```python
from build123d import *

# Parameters (mm, degrees)
EXTRUDE_1_DEPTH = 50
SHELL_1_T       = -5
EXTRUDE_3_DEPTH = 45


with BuildPart() as part:
    # 스케치1 → 보스-돌출1 (new body)
    with BuildSketch(Plane(origin=(0, 0, 0), x_dir=(1, 0, 0), z_dir=(0, 1, 0))):
        with BuildLine():
            Line((10, 0), (270, 0))
            ThreePointArc((270, 0), (277.071067812, 2.928932188), (280, 10))
            Line((280, 10), (280, 220))
            ThreePointArc((280, 220), (277.071067812, 227.071067812), (270, 230))
            Line((270, 230), (10, 230))
            ThreePointArc((10, 230), (2.928932188, 227.071067812), (0, 220))
            Line((0, 220), (0, 10))
            ThreePointArc((0, 10), (2.928932188, 2.928932188), (10, 0))
        make_face()
    extrude(amount=EXTRUDE_1_DEPTH)

    # 쉘1
    shell_1_openings = [part.faces().sort_by_distance(p)[0] for p in [
        (140, 50, -115),
    ]]
    offset(amount=SHELL_1_T, openings=shell_1_openings, kind=Kind.INTERSECTION)

    # 스케치4 → 보스-돌출3 (add)
    with BuildSketch(Plane(origin=(0, 5, 0), x_dir=(1, 0, 0), z_dir=(0, 1, 0))):
        Polygon((5, 117.5), (5, 112.5), (92.5, 112.5), (92.5, 5), (97.5, 5), (97.5, 112.5), (180, 112.5), (180, 5), (185, 5), (185, 112.5), (275, 112.5), (275, 117.5), (185, 117.5), (185, 225), (180, 225), (180, 117.5), (97.5, 117.5), (97.5, 225), (92.5, 225), (92.5, 117.5), align=None)
    extrude(amount=EXTRUDE_3_DEPTH)


solid = part.part
```
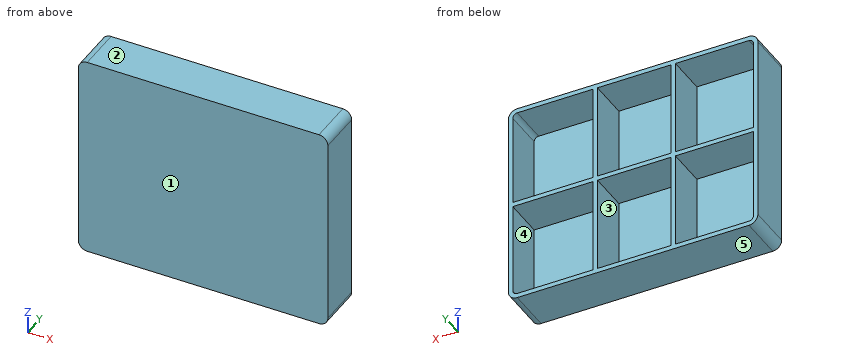
Could you check a few things on this model? Use its own coordinates, in mm. Face numbers are marked on the shaded views. A direction names the side the tool comes from. Round coordinates to 2 decimals unless told otherwise and drop trailing zeros. Order: outer loops, then holes, each group sorted by start corner. A loop starts at its lowest first (then second) coordinate and runs counter-clockwise, first axis right, second up. Notation, with made-up numbers: (-38.5, 23) -> (13.5, 23) arc R12 ccw to (13.5, 37) -> close; hole circle Ø1 at (29, 55). An arc over 180 degrees is marked (long way). One line per question, with ' | ' between items.
Q1. Which directions (+Z, -Z, +X, -X, +Y, -Y) give clear straight access to the entire face, cutting with the end or side of a thin tool? Please do the marked faces 4 and 5.
Computed values:
face 4: +Y | face 5: -Z, +X, -X, +Y, -Y
Q2. If I drill on line 1 (X direction, y = 13, z = -218); line 2 (Z direction, x = 176.5, y = 22.5); line 3 (Y direction, x = 130.5, z = -208), over which ranges is the centre line in solid material (lowest first)? Write a range as from..to.
Computed values:
line 1: 0..5, 92.5..97.5, 180..185, 275..280 | line 2: -230..-225, -117.5..-112.5, -5..0 | line 3: 0..5
Q3. If we section it at B-B on x = 154.5: Write out the boundary of the cut face in (y, z), plus the area to 4 significant figures.
Computed values:
outline: (0, -230) -> (50, -230) -> (50, -225) -> (5, -225) -> (5, -117.5) -> (50, -117.5) -> (50, -112.5) -> (5, -112.5) -> (5, -5) -> (50, -5) -> (50, 0) -> (0, 0) -> close | area: 1,825 mm²
Q4. I'm going to push flat-ended pins straight in: pin 1 (4 mm diameter, centred on x = 81, z = -104.5, fed in from -Y); pin 2 (6 mm diameter, centred on x = 212.5, z = -75.5, fed in from +Y). Where does each tip first touch, or does it pass through?
Computed values:
pin 1: y = 0 | pin 2: y = 5
Q5. If we section it at A-A on z = -138.5: Write out the boundary of the cut face in (x, y), plus the area to 3 significant figures.
Computed values:
outline: (0, 0) -> (280, 0) -> (280, 50) -> (275, 50) -> (275, 5) -> (185, 5) -> (185, 50) -> (180, 50) -> (180, 5) -> (97.5, 5) -> (97.5, 50) -> (92.5, 50) -> (92.5, 5) -> (5, 5) -> (5, 50) -> (0, 50) -> close | area: 2,300 mm²
Q6. If we section it at C-C on y = 14.5: Give the number of separate pieces and of enclosed holes in the cut face, plus the area to 3 significant figures.
Computed values:
separate pieces: 1 | enclosed holes: 6 | area: 8,440 mm²
Q7. We'd pull the mould along Z, two halves only. Please class the marked faces 1, 2 and 3: released by +Z, released by -Z, zero draft, split by the parting line, or undercut.
Computed values:
face 1: zero draft | face 2: released by +Z | face 3: undercut
